Design review of the part shown in the three views and the two pictorial views. Dimensions are in mm from the part's minimum x, y and z. A direction names the side the tool comes from. Give positions to 0.01 mm unless a question says otherwise; leave off trailing zeros. Order: outer loops, then holes, each group sorted by start corner. A loop starts at its lowest first (then second) coordinate and runs counter-clockwise, first axis right, second up.
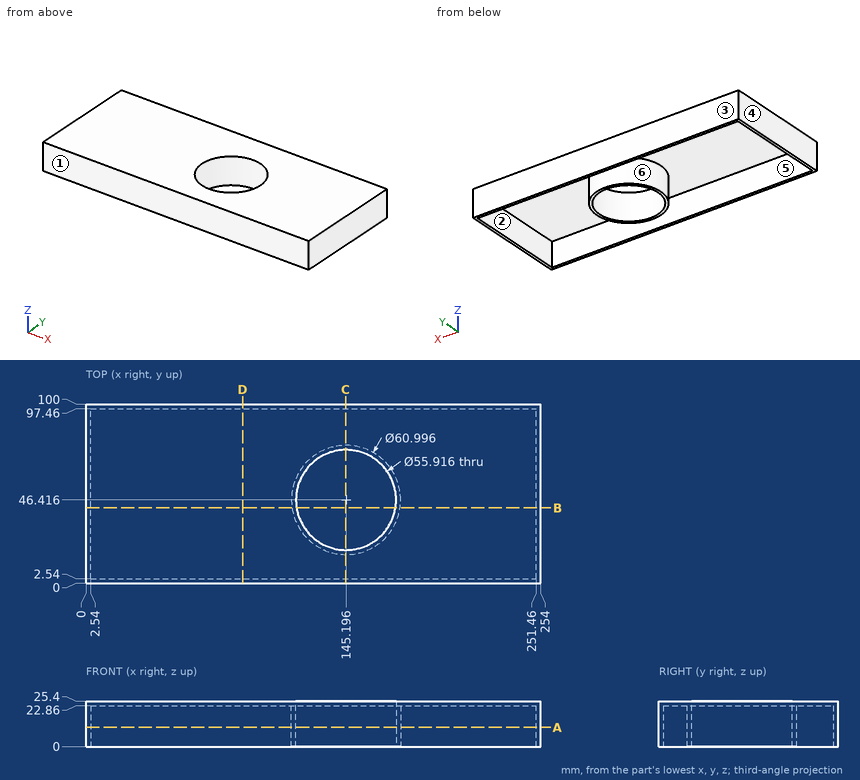
1) Draft analysis for pull direction X (two halves, no side actions). For the marked faces 3, 4, 5 and 6, state which applies: +X half, -X half, draft (parallel to the pull), parting line (faces both ways), or undercut.
Answer sheet:
face 3: draft
face 4: -X half
face 5: undercut
face 6: undercut
2) We need section D-D on x = 87.5. Give the boundary of the cut face in (y, z), then the cut area to 3 significant figures.
Answer sheet:
outline: (0, 0) - (2.54, 0) - (2.54, 22.86) - (97.46, 22.86) - (97.46, 0) - (100, 0) - (100, 25.4) - (0, 25.4) - close
area: 370 mm2
3) Clearance check with a flat-ended pin moving along its axis: pin 1 (1 mm diameter, centred on x = 187.5, y = 83, fed in from -Z). State where the tip first meets the part, or that it passes through.
Answer sheet:
pin 1: stops at z = 22.86
4) We need section A-A on z = 10.75. Give the boundary of the cut face in (x, y).
Answer sheet:
outline: (0, 0) - (254, 0) - (254, 100) - (0, 100) - close; circle Ø61 at (145.2, 46.42); hole (2.54, 2.54) - (251.46, 2.54) - (251.46, 97.46) - (2.54, 97.46) - close; hole circle Ø55.92 at (145.2, 46.42)
5) To check wall thickness, follow line 1 (Y direction, x = 32, z = 18); line 2 (X direction, y = 53, z = 20.5) (1 decimal); line 3 (X direction, y = 15, z = 4). State the ranges of each line that lie inside material, in increasing order.
Answer sheet:
line 1: y = 0 to 2.54, 97.46 to 100
line 2: x = 0 to 2.5, 115.4 to 118, 172.4 to 175, 251.5 to 254
line 3: x = 0 to 2.54, 251.46 to 254
6) We need section B-B on y = 42. Give the boundary of the cut face in (x, z).
Answer sheet:
outline: (0, 0) - (2.54, 0) - (2.54, 22.86) - (115.02, 22.86) - (115.02, 0) - (117.59, 0) - (117.59, 25.4) - (0, 25.4) - close; (172.8, 0) - (175.37, 0) - (175.37, 22.86) - (251.46, 22.86) - (251.46, 0) - (254, 0) - (254, 25.4) - (172.8, 25.4) - close
7) Tool access review of the marked faces 1 and 2: name each direction out of +Z, -Z, +X, -X, +Y, -Y from which nothing blocks a thin tool from reaching the whole face with its end or side.
Answer sheet:
face 1: +Z, -Z, +X, -X, -Y
face 2: -Z
8) We need section C-C on x = 145. Give the boundary of the cut face in (y, z).
Answer sheet:
outline: (0, 0) - (2.54, 0) - (2.54, 22.86) - (15.92, 22.86) - (15.92, 0) - (18.46, 0) - (18.46, 25.4) - (0, 25.4) - close; (74.37, 0) - (76.91, 0) - (76.91, 22.86) - (97.46, 22.86) - (97.46, 0) - (100, 0) - (100, 25.4) - (74.37, 25.4) - close
